from build123d import *

# Parameters (mm, degrees)
F0_W     = 100
F0_H     = 100
F1_DEPTH = 40
F2_T     = -2.5
F3_R     = 1.2
F4_DEPTH = 97.501
F5_DEPTH = 25
F6_R     = 1
F7_DEPTH = 25


with BuildPart() as f1:
    # F0 (on Top) → F1 (new body)
    with BuildSketch(Plane.XY):
        Rectangle(F0_W, F0_H)
    extrude(amount=F1_DEPTH)

    # F2
    f2_openings = [f1.faces().sort_by_distance(p)[0] for p in [
        (0, 0, 40),
    ]]
    offset(amount=F2_T, openings=f2_openings)

    # F3 (on face) → F4 (cut, through all)
    with BuildSketch(Plane(origin=(47.5, 0, 0), x_dir=(0, -1, 0), z_dir=(-1, 0, 0))):
        with Locations((0, 16.35)):
            Circle(F3_R)
    extrude(amount=F4_DEPTH, mode=Mode.SUBTRACT)

    # F3 (on face) → F5 (cut)
    with BuildSketch(Plane(origin=(47.5, 0, 0), x_dir=(0, -1, 0), z_dir=(-1, 0, 0))):
        with Locations((0, 16.35)):
            Circle(F3_R)
    extrude(amount=-F5_DEPTH, mode=Mode.SUBTRACT)

    # F6 (on face) → F7 (cut)
    with BuildSketch(Plane.XY.offset(2.5)):
        with Locations((-17.5, -8.5)):
            Circle(F6_R)
        with Locations((17.5, -8.5)):
            Circle(F6_R)
        with Locations((17.5, 45.5)):
            Circle(F6_R)
        with Locations((-17.5, 45.5)):
            Circle(F6_R)
    extrude(amount=-F7_DEPTH, mode=Mode.SUBTRACT)


solid = f1.part
Geometry: final body of the model. Coordinates: model frame, mm. A direction names the side the tool comes from. Round coordinates to 2 decimals unless told otherwise and drop trailing zeros. Loops run counter-clockwise (first coordinate to the right, second up) from the corner with the lowest first, then second, coordinate; pieces in that order, holes last.
Q1. Pull-direction query (X, two-part tool) for faces 3 (the flat face through (-1, -47.5, 21)), 4 (the flat face through (-1, 50, 20)), 5 (the flat face through (-50, -1, 20)); classes: released by +X, released by -X, zero draft, split by the parting line, or undercut.
Q2. Section D-D on x = 8.5. Return loops of the section in (y, z).
Q3. Section C-C on z = 16.35. Return loops of the section in (x, y).
Q4. Section A-A on y = 0. Return loops of the section in (x, z).
Q5. Section B-B on z = 30.5. Return loops of the section in (x, y), plus the area to 3 significant figures.
Q6. Pin query (flat end, axial travel): P1, Ø2, axis at y = 0, z = 16.35, coming from the -X side; P2, Ø2.5, axis at x = 17.5, y = 45.5, coming from the +Z side. Return the tip coordinate at first contact, or that it passes through.
Q7. Material intervals for L1, parallel to Y at x = 17.5, z = 1.8; L2, parallel to Y at x = -13, z = 21, sorted ascending.
Q8. Access query for faces 1 (the flat face through (-1, 1, 2.5)), 2 (the cylindrical face through (-48.73, 0.16, 17.54)). Directions: +Z, -Z, +X, -X, +Y, -Y. A direction counts if a zero-diameter tool reaches every point of the face in a straight line with its end or side. Return the directions, or none.
Evaluation:
1. face 3: undercut
1. face 4: zero draft
1. face 5: released by -X
2. outline: (-50, 0) - (50, 0) - (50, 40) - (47.5, 40) - (47.5, 2.5) - (-47.5, 2.5) - (-47.5, 40) - (-50, 40) - close
3. outline: (-50, -50) - (50, -50) - (50, -1.2) - (47.5, -1.2) - (47.5, -47.5) - (-47.5, -47.5) - (-47.5, -1.2) - (-50, -1.2) - close; (-50, 1.2) - (-47.5, 1.2) - (-47.5, 47.5) - (47.5, 47.5) - (47.5, 1.2) - (50, 1.2) - (50, 50) - (-50, 50) - close
4. outline: (-50, 0) - (50, 0) - (50, 15.15) - (47.5, 15.15) - (47.5, 2.5) - (-47.5, 2.5) - (-47.5, 15.15) - (-50, 15.15) - close; (-50, 17.55) - (-47.5, 17.55) - (-47.5, 40) - (-50, 40) - close; (47.5, 17.55) - (50, 17.55) - (50, 40) - (47.5, 40) - close
5. outline: (-50, -50) - (50, -50) - (50, 50) - (-50, 50) - close; hole (-47.5, -47.5) - (47.5, -47.5) - (47.5, 47.5) - (-47.5, 47.5) - close
5. area: 975 mm2
6. P1: passes through
6. P2: stops at z = 2.5
7. L1: y = -50 to -9.5, -7.5 to 44.5, 46.5 to 50
7. L2: y = -50 to -47.5, 47.5 to 50
8. face 1: +Z
8. face 2: +X, -X
